Check sheet for the drawn part. Datum: minimum x, y, z corner. Units: mm. Give positions to 0.01 mm unless a question says otherwise; leave off trailing zeros. Write each loop counter-clockwise with the first axis right and the second up, starting at its lowest first coordinate (ties: lowest second). Pieces come first, ordered by that corner, then holes.
(1) Cross-section at B-B (z = 17.5). Record the boundary of the cut face in (x, y).
(2) Thickness scan on line 1 along X through (y, z) = (2.1, 17.5); line 2 along Z through (x, y) = (17, 1.85); line 3 along Z through (x, y) = (19.5, 1). Record the ranges inside material, lowest first.
(3) Depth check by flat-ended pin: P1, Ø1.5, axis at x = 6.5, y = 3, coming from the -Z side (1 decimal); P2, Ø6.5, axis at x = 17.5, z = 17.5, coming from the -Y side; P3, Ø3, axis at y = 2, z = 12.5, coming from the +X side. Enter the tip coordinate at first touch or a pass-through.
(4) Cross-section at D-D (y = 4.25). Record the boundary of the cut face in (x, z).
(5) Cross-section at A-A (x = 17.5). Record the boundary of the cut face in (y, z), and give its area (3 significant figures).
(6) Mould release check, pull along Y, two halves, no side actions. Record for the marked faces 1, 2 and 3: +Y half, -Y half, draft (parallel to the pull), parting line (faces both ways), or undercut.
(7) Cross-section at C-C (y = 2.05). Record the boundary of the cut face in (x, z).
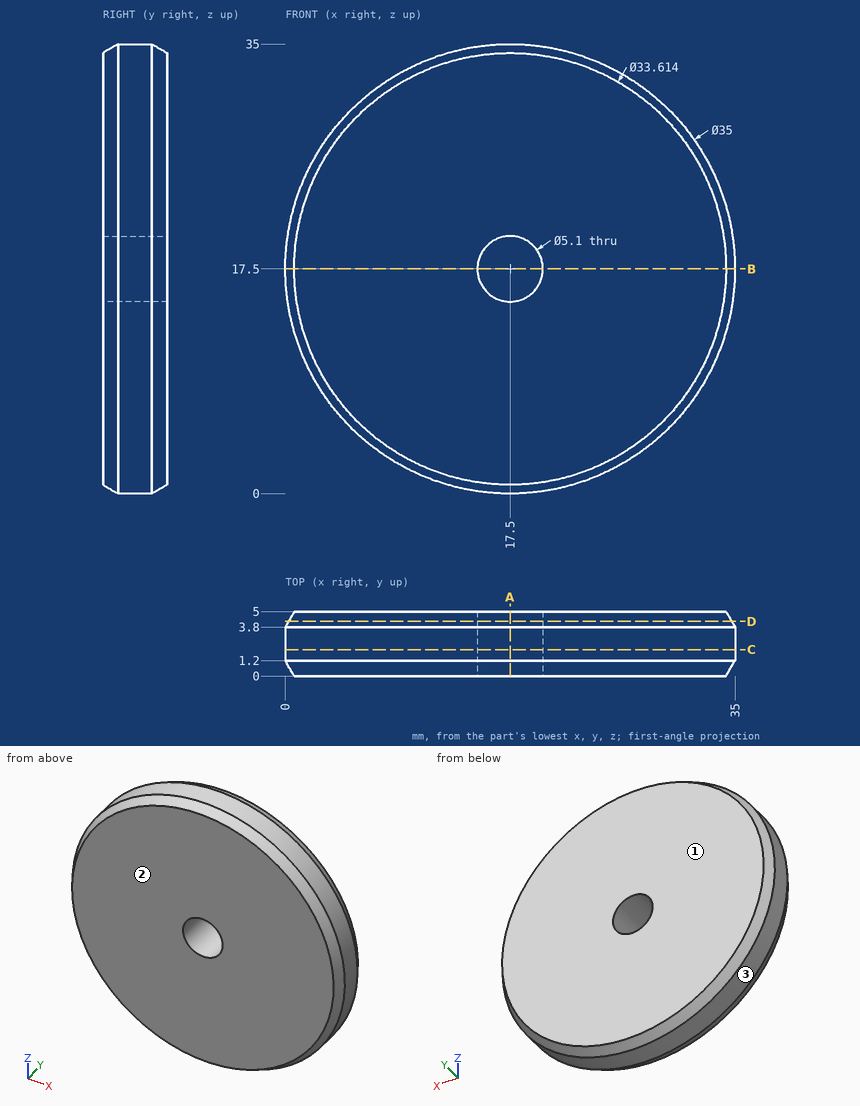
Reply:
1. outline: (0, 1.2) - (0.69, 0) - (14.95, 0) - (14.95, 5) - (0.69, 5) - (0, 3.8) - close; (20.05, 0) - (34.31, 0) - (35, 1.2) - (35, 3.8) - (34.31, 5) - (20.05, 5) - close
2. line 1: x = 0 to 14.95, 20.05 to 35
2. line 2: z = 0.01 to 15, 20 to 34.99
2. line 3: z = 0.23 to 15.92, 19.08 to 34.77
3. P1: stops at z = 3.3
3. P2: stops at y = 0
3. P3: stops at x = 34.65
4. outline: circle Ø34.48 at (17.5, 17.5); hole circle Ø5.1 at (17.5, 17.5)
5. outline: (0, 0.69) - (1.2, 0) - (3.8, 0) - (5, 0.69) - (5, 14.95) - (0, 14.95) - close; (0, 20.05) - (5, 20.05) - (5, 34.31) - (3.8, 35) - (1.2, 35) - (0, 34.31) - close
5. area: 148 mm2
6. face 1: +Y half
6. face 2: -Y half
6. face 3: draft
7. outline: circle Ø35 at (17.5, 17.5); hole circle Ø5.1 at (17.5, 17.5)
